Check sheet for the modelled part. Datum: model origin and axes. Units: mm. Face numbers are marked on the shaded views. A direction names the side the tool comes from. Give positions to 0.01 mm unless a question says otherwise; leave off trailing zeros. Order: outer loops, then holes, each group sorted by start corner. A loop starts at its lowest first (then second) coordinate and runs counter-clockwise, first axis right, second up. Notation, with made-up numbers: (-22, 7.25) -> (2, 7.25) arc R27 ccw to (2, 34.25) -> close; hole circle Ø11 at (-40, 40). An arc over 180 degrees is marked (long way). Answer in a Markdown table with one row per item. Add a question column.
(1) Cross-section at B-B (x = -3). Record the cut outline in (y, z).
(2) Release check for a two-part mould opening along Y. For the marked faces 6, 7 and 8 record: released by +Y, released by -Y, zero draft, split by the parting line, or undercut.
(3) Cross-section at A-A (y = 25). Record the cut outline in (x, z).
(4) Cross-section at C-C (y = 15.5). Record the cut outline in (x, z), then the cut area to 3 significant figures.
(5) Go/stop test with flat-tipped pins: pin 1 (3 mm diameter, centred on x = 16, y = -17, fed in from +Z); pin 2 (8 mm diameter, centred on y = 23, z = 10.5, fed in from -X); pin 3 (6 mm diameter, centred on x = 8.5, y = -16, fed in from +Z); pin 4 (7 mm diameter, centred on x = 11.5, y = -6, fed in from +Z). Record where each tip stops, or that it passes through.
(6) Cross-section at D-D (x = -22). Record the cut outline in (y, z), then the cut area to 3 significant figures.
(7) Set-up check for the marked faces 1, 2, 3, 4 and 5: record each of +Z, -Z, +X, -X, +Y, -Y from which the full face is reachable in a straight line by a thin tool's end or side.
(8) Thickness scan on L1, parallel to Y at x = -24.7, z = 10; L2, parallel to Y at x = -0.5, z = 6; L3, parallel to X at y = -16.5, z = 14.75. Record the ranges inside material, lowest first. Write a range as [from, to].
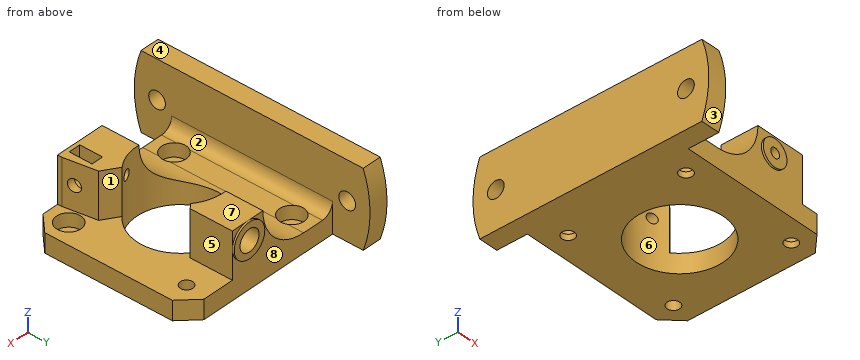
```python
from build123d import *

# Parameters (mm, degrees)
SKETCH1_W               = 42.3
SKETCH1_H               = 42.3
BOSS_EXTRUDE1_DEPTH     = 5
CHAMFER1_SIZE           = 4.38
SKETCH4_W               = 5
SKETCH4_H               = 62
BOSS_EXTRUDE2_DEPTH     = 20
SKETCH5_R               = 2.2
CUT_EXTRUDE3_DEPTH      = 60.985748307
BOSS_EXTRUDE3_DEPTH     = 42.3
FILLET1_R               = 3
CUT_EXTRUDE1_DEPTH      = 44.24144424
CUT_EXTRUDE1_DEPTH_BACK = 44.24144424
SKETCH2_R               = 11.433895
SKETCH2_R_2             = 1.65
CUT_EXTRUDE2_DEPTH      = 44.24144424
CUT_EXTRUDE2_DEPTH_BACK = 3.5
SKETCH3_R               = 3.2
SKETCH7_R               = 1.27442
CUT_EXTRUDE4_DEPTH      = 62.672076339
BOSS_EXTRUDE4_START     = 0.5
SKETCH8_R               = 3.5
SKETCH8_R_2             = 1.27442
BOSS_EXTRUDE4_DEPTH     = 0.5
SKETCH9_R               = 2.8
CUT_EXTRUDE5_DEPTH      = 4
BOSS_EXTRUDE5_START     = 0.5
SKETCH10_R              = 4.5
SKETCH10_R_2            = 2.8
BOSS_EXTRUDE5_DEPTH     = 0.5
SKETCH11_W              = 3.1
SKETCH11_H              = 6
CUT_EXTRUDE6_DEPTH      = 7.826
CUT_EXTRUDE7_DEPTH      = 50.648434779
CUT_EXTRUDE7_DEPTH_BACK = 0.45
SKETCH12_R              = 1.62
CUT_EXTRUDE8_REACH      = 45.975


with BuildPart() as part:
    # Sketch1 → Boss-Extrude1 (new body)
    with BuildSketch(Plane.XY):
        Rectangle(SKETCH1_W, SKETCH1_H)
    extrude(amount=BOSS_EXTRUDE1_DEPTH)

    # Chamfer1
    chamfer1_edges = [part.edges().sort_by_distance(p)[0] for p in [
        (21.15, -21.15, 2.5),
        (21.15, 21.15, 2.5),
    ]]
    chamfer(chamfer1_edges, length=CHAMFER1_SIZE)

    # Sketch4 → Boss-Extrude2 (add)
    with BuildSketch(Plane(origin=(0, 0, 0), x_dir=(-1, 0, 0), z_dir=(0, 0, -1))):
        with Locations((23.65, 0)):
            Rectangle(SKETCH4_W, SKETCH4_H)
    extrude(amount=-BOSS_EXTRUDE2_DEPTH)

    # Sketch5 → Cut-Extrude3 (cut, through all)
    with BuildSketch(Plane.ZY.offset(26.15)):
        with Locations((10, 25)):
            Circle(SKETCH5_R)
        with Locations((10, -25)):
            Circle(SKETCH5_R)
        with BuildLine():
            Line((0, 29.205999997), (0, 32.205999997))
            Line((0, 32.205999997), (20, 32.205999997))
            Line((20, 32.205999997), (20, 29.205999997))
            ThreePointArc((20, 29.205999997), (10, 31), (0, 29.205999997))
        make_face()
        with BuildLine():
            Line((20, -29.205999997), (20, -32.205999997))
            Line((20, -32.205999997), (0, -32.205999997))
            Line((0, -32.205999997), (0, -29.205999997))
            ThreePointArc((0, -29.205999997), (10, -31), (20, -29.205999997))
        make_face()
    extrude(amount=-CUT_EXTRUDE3_DEPTH, mode=Mode.SUBTRACT)

    # Sketch6 → Boss-Extrude3 (add)
    with BuildSketch(Plane.XZ.offset(21.15)):
        with BuildLine():
            Line((12.462, 5), (12.462, 17))
            Line((12.462, 17), (-0.624, 17))
            ThreePointArc((-0.624, 17), (-4.138718626, 8.514718626), (-12.624, 5))
            Line((-12.624, 5), (12.462, 5))
        make_face()
    extrude(amount=-BOSS_EXTRUDE3_DEPTH)

    # Fillet1
    fillet1_edges = [part.edges().sort_by_distance(p)[0] for p in [
        (-21.15, 0, 5),
    ]]
    fillet(fillet1_edges, radius=FILLET1_R)

    # Sketch2 → Cut-Extrude1 (cut, two sides: drawn at the far end of the back side and taken through both)
    with BuildSketch(Plane.XY.offset(5).offset(-CUT_EXTRUDE1_DEPTH_BACK)):
        with Locations(Location((0.01611, 0, 0), (0, 0, 266.790701126))):
            Circle(SKETCH2_R)
        with Locations(Location((-15.48389, 15.5, 0), (0, 0, 180))):
            Circle(SKETCH2_R_2)
        with Locations(Location((15.51611, 15.5, 0), (0, 0, 180))):
            Circle(SKETCH2_R_2)
        with Locations(Location((15.51611, -15.5, 0), (0, 0, 180))):
            Circle(SKETCH2_R_2)
        with Locations(Location((-15.48389, -15.5, 0), (0, 0, 180))):
            Circle(SKETCH2_R_2)
    extrude(amount=CUT_EXTRUDE1_DEPTH + CUT_EXTRUDE1_DEPTH_BACK, mode=Mode.SUBTRACT)

    # Sketch3 → Cut-Extrude2 (cut, two sides: drawn at the far end of the back side and taken through both)
    with BuildSketch(Plane.XY.offset(5).offset(-CUT_EXTRUDE2_DEPTH_BACK)):
        with Locations(Location((-15.48389, 15.5, 0), (0, 0, 213.57533661))):
            Circle(SKETCH3_R)
        with Locations(Location((-15.48389, -15.5, 0), (0, 0, 213.57533661))):
            Circle(SKETCH3_R)
        with Locations(Location((15.51611, -15.5, 0), (0, 0, 197.367581673))):
            Circle(SKETCH3_R)
    extrude(amount=CUT_EXTRUDE2_DEPTH + CUT_EXTRUDE2_DEPTH_BACK, mode=Mode.SUBTRACT)

    # Sketch7 → Cut-Extrude4 (cut, through all)
    with BuildSketch(Plane.XZ.offset(21.15)):
        with Locations(Location((3.87669, 12.5, 0), (0, 0, 270))):
            Circle(SKETCH7_R)
    extrude(amount=-CUT_EXTRUDE4_DEPTH, mode=Mode.SUBTRACT)

    # Sketch8 → Boss-Extrude4 (add)
    with BuildSketch(Plane.XZ.offset(21.15).offset(BOSS_EXTRUDE4_START)):
        with Locations(Location((3.87669, 12.5, 0), (0, 0, 90))):
            Circle(SKETCH8_R)
        with Locations(Location((3.87669, 12.5, 0), (0, 0, 270))):
            Circle(SKETCH8_R_2, mode=Mode.SUBTRACT)
    extrude(amount=-BOSS_EXTRUDE4_DEPTH)

    # Sketch9 → Cut-Extrude5 (cut)
    with BuildSketch(Plane(origin=(0, 21.15, 0), x_dir=(1, 0, 0), z_dir=(0, 1, 0))):
        with Locations(Location((3.87669, -12.5, 0), (0, 0, 270))):
            Circle(SKETCH9_R)
    extrude(amount=-CUT_EXTRUDE5_DEPTH, mode=Mode.SUBTRACT)

    # Sketch10 → Boss-Extrude5 (add)
    with BuildSketch(Plane(origin=(0, 21.15, 0), x_dir=(1, 0, 0), z_dir=(0, 1, 0)).offset(BOSS_EXTRUDE5_START)):
        with Locations(Location((3.87669, -12.5, 0), (0, 0, 270))):
            Circle(SKETCH10_R)
        with Locations(Location((3.87669, -12.5, 0), (0, 0, 270))):
            Circle(SKETCH10_R_2, mode=Mode.SUBTRACT)
    extrude(amount=-BOSS_EXTRUDE5_DEPTH)

    # Sketch11 → Cut-Extrude6 (cut)
    with BuildSketch(Plane.XY.offset(17)):
        with Locations((8.626, -17.15)):
            Rectangle(SKETCH11_W, SKETCH11_H)
    extrude(amount=-CUT_EXTRUDE6_DEPTH, mode=Mode.SUBTRACT)

    # Sketch12 → Cut-Extrude7 (cut, two sides: drawn at the far end of the back side and taken through both)
    with BuildSketch(Plane(origin=(7.076, 0, 0), x_dir=(0, 0, -1), z_dir=(1, 0, 0)).offset(-CUT_EXTRUDE7_DEPTH_BACK)):
        with Locations(Location((-11.25, -17.15, 0), (0, 0, 154.603036972))):
            Circle(SKETCH12_R)
    extrude(amount=CUT_EXTRUDE7_DEPTH + CUT_EXTRUDE7_DEPTH_BACK, mode=Mode.SUBTRACT)

    # Cut-Extrude8: up to this face of the body (flat: up to its plane)
    cut_extrude8_end = Plane(part.part.faces().sort_by_distance((16.794233337, 1.179955887, 5))[0])
    # Sketch13 → Cut-Extrude8 (cut, up to the picked face)
    with BuildSketch(Plane.XY.offset(17), mode=Mode.PRIVATE) as cut_extrude8_sk1:
        with BuildLine():
            Line((12.462, 21.15), (8.37669, 21.15))
            Line((8.37669, 21.15), (8.37669, 10.042))
            Line((8.37669, 10.042), (7.05269, 9.012241496))
            ThreePointArc((7.05269, 9.012241496), (11.450004992, -0.000437691), (7.052, -9.012780191))
            Line((7.052, -9.012780191), (11.082, -11.582))
            Line((11.082, -11.582), (12.462, -20))
            Line((12.462, -20), (12.462, 21.15))
        make_face()
    cut_extrude8_tool1 = split(extrude(cut_extrude8_sk1.sketch, amount=-CUT_EXTRUDE8_REACH, mode=Mode.PRIVATE), bisect_by=cut_extrude8_end, keep=Keep.BOTH, mode=Mode.PRIVATE)
    add(cut_extrude8_tool1.solids().sort_by(Axis((10.711689, 5.447253, 17), (0, 0, -1)))[0], mode=Mode.SUBTRACT)


solid = part.part
```
Answer below:
| question | item | result |
|---|---|---|
| 1 | outline | (-21.15, 0) -> (-11.03, 0) -> (-11.03, 9.83) -> (-21.15, 9.83) -> close; (11.03, 0) -> (21.15, 0) -> (21.15, 9.83) -> (11.03, 9.83) -> close |
| 2 | face 6 | undercut |
| 2 | face 7 | zero draft |
| 2 | face 8 | released by +Y |
| 3 | outline | (-26.15, 0) -> (-21.15, 0) -> (-21.15, 7.8) -> (-26.15, 7.8) -> close; (-26.15, 12.2) -> (-21.15, 12.2) -> (-21.15, 20) -> (-26.15, 20) -> close |
| 4 | outline | (-26.15, 0) -> (-17.13, 0) -> (-17.13, 1.5) -> (-18.68, 1.5) -> (-18.68, 5.05) arc R3 cw to (-21.15, 8) -> (-21.15, 20) -> (-26.15, 20) -> close; (-13.83, 0) -> (13.87, 0) -> (13.87, 5) -> (8.38, 5) -> (8.38, 17) -> (-0.62, 17) arc R12 cw to (-12.28, 5) -> (-12.28, 1.5) -> (-13.83, 1.5) -> close; (17.17, 0) -> (21.15, 0) -> (21.15, 5) -> (17.17, 5) -> close; hole circle Ø2.55 at (3.88, 12.5) |
| 4 | area | 403 mm² |
| 5 | pin 1 | stops at z = 1.5 |
| 5 | pin 2 | stops at x = -26.15 |
| 5 | pin 3 | stops at z = 17 |
| 5 | pin 4 | stops at z = 5 |
| 6 | outline | (-29.21, 0) -> (29.21, 0) arc R28.77 ccw to (29.21, 20) -> (-29.21, 20) arc R28.77 ccw to start; hole circle Ø4.4 at (-25, 10); hole circle Ø4.4 at (25, 10) |
| 6 | area | 1,190 mm² |
| 7 | face 1 | +Z, +X |
| 7 | face 2 | +Z, +Y, -Y |
| 7 | face 3 | +X, -X, -Y |
| 7 | face 4 | +Z, +X, -X, +Y, -Y |
| 7 | face 5 | +Z, +X, +Y |
| 8 | L1 | y = [-31, -27.2], [-22.8, 22.8], [27.2, 31] |
| 8 | L2 | y = [-21.15, -11.42], [11.42, 21.15] |
| 8 | L3 | x = [-26.15, -21.15], [-0.84, 7.08], [10.18, 11.89] |
